Input: part model. Units: mm. Frame: model coordinates. A direction names the side the tool comes from. Coordinates: 2 decimals unless noted, no trailing zeros. Write each loop counter-clockwise with the first axis right and the second up, starting at its lowest first coordinate (ties: lowest second). Pieces come first, ordered by that corner, then holes. Notation, with made-up numbers: (9, 42) - (33, 42) arc R14 cw to (33, 68) - close; hole circle Ø5 at (85, -23). An arc over 180 degrees is marked (long way). Use a Markdown table: item, result. Add a question column.
Q1. Section query A-A (x = 0). Return the cut outline in (y, z) (1 decimal).
Q2. Section query D-D (x = -23). Return the cut outline in (y, z) (3 decimals).
Q3. Section query C-C (y = 50.8). Return the cut outline in (x, z) (1 decimal).
Q4. Set-up query: faces 1 (the face through (13.025, 32.07, 4.696)), 2 (the face through (-45.3, 45.4, 4.7)). Return all of +Z, -Z, +X, -X, +Y, -Y with unobstructed straight access to the full face (end or side cutting, diameter ignored); none if empty.
Q5. Mould query, pull axis X, two halves, no side actions, for faces 3 (the face through (23.315, 55.576, 4.696)), 4 (the face through (-25.72, 25.65, 4.83)), 5 (the face through (-22.812, 55.785, 4.696)). Classes: released by +X, released by -X, zero draft, split by the parting line, or undercut.
Q6. Section query B-B (z = 1.25). Return the cut outline in (x, y) (1 decimal), then the cut area to 3 significant figures.
Q7. Material intervals for probe 1 along Y at (x, z) = (0, 4.5) (1 decimal); probe 2 along X at (y, z) = (-2, 7.25); probe 3 along X at (y, z) = (-3.5, 3.5), sorted ascending. Write a range as from..to.
Q8. Pin query (flat end, axial travel): P1, Ø10, axis at x = 46, y = 6.5, coming from the -Z side; P2, Ø4, axis at x = 17.5, z = 8.5, coming from the +Y side; P3, Ø1.5, axis at x = 10.5, z = 3.5, coming from the +Y side; P4, Ø8.5, axis at x = 0, y = 50.8, coming from the +Z side. Return the tip coordinate at first contact, or that it passes through.
from build123d import *

# Parameters (mm, degrees)
F0_R     = 4.7625
F1_DEPTH = 9.525
F2_R     = 12.7635


with BuildPart() as f1:
    # F0 (on Top) → F1 (new body)
    with BuildSketch(Plane.XY):
        with BuildLine():
            ThreePointArc((-38.331487, -4.728468), (-37.68341, -2.403602), (-37.465, 0))
            ThreePointArc((-37.465, 0), (-48.198471, 13.078772), (-63.119934, 5.103084))
            ThreePointArc((-63.119934, 5.103084), (-55.716337, -12.395638), (-38.331487, -4.728468))
        make_face()
        with Locations((-50.8, 0)):
            Circle(F0_R, mode=Mode.SUBTRACT)
        with BuildLine():
            ThreePointArc((-63.119934, 5.103084), (-48.198471, 13.078772), (-37.465, 0))
            ThreePointArc((-37.465, 0), (-37.68341, -2.403602), (-38.331487, -4.728468))
            Line((-38.331487, -4.728468), (-26.491756, 26.491756))
            ThreePointArc((-26.491756, 26.491756), (-43.329554, 24.833377), (-48.240958, 41.024108))
            Line((-48.240958, 41.024108), (-63.119934, 5.103084))
        make_face()
        with BuildLine():
            ThreePointArc((-41.024108, 48.240958), (-45.350293, 45.350293), (-48.240958, 41.024108))
            ThreePointArc((-48.240958, 41.024108), (-43.329554, 24.833377), (-26.491756, 26.491756))
            ThreePointArc((-26.491756, 26.491756), (-23.601091, 30.817941), (-22.586024, 35.921024))
            ThreePointArc((-22.586024, 35.921024), (-28.512495, 47.008672), (-41.024108, 48.240958))
        make_face()
        with BuildLine():
            ThreePointArc((-22.586024, 35.921024), (-23.601091, 30.817941), (-26.491756, 26.491756))
            Line((-26.491756, 26.491756), (0, 37.465))
            ThreePointArc((0, 37.465), (-13.078772, 48.198471), (-5.103084, 63.119934))
            Line((-5.103084, 63.119934), (-41.024108, 48.240958))
            ThreePointArc((-41.024108, 48.240958), (-28.512495, 47.008672), (-22.586024, 35.921024))
        make_face()
        with BuildLine():
            ThreePointArc((-5.103084, 63.119934), (-13.078772, 48.198471), (0, 37.465))
            ThreePointArc((0, 37.465), (9.429269, 41.370731), (13.335, 50.8))
            ThreePointArc((13.335, 50.8), (11.087647, 58.208529), (5.103084, 63.119934))
            ThreePointArc((5.103084, 63.119934), (0, 64.135), (-5.103084, 63.119934))
        make_face()
        with Locations((0, 50.8)):
            Circle(F0_R, mode=Mode.SUBTRACT)
        with BuildLine():
            ThreePointArc((13.335, 50.8), (9.429269, 41.370731), (0, 37.465))
            Line((0, 37.465), (26.491756, 26.491756))
            ThreePointArc((26.491756, 26.491756), (24.833377, 43.329554), (41.024108, 48.240958))
            Line((41.024108, 48.240958), (5.103084, 63.119934))
            ThreePointArc((5.103084, 63.119934), (11.087647, 58.208529), (13.335, 50.8))
        make_face()
        with BuildLine():
            ThreePointArc((41.024108, 48.240958), (24.833377, 43.329554), (26.491756, 26.491756))
            ThreePointArc((26.491756, 26.491756), (41.024108, 23.601091), (49.256024, 35.921024))
            ThreePointArc((49.256024, 35.921024), (48.999796, 38.522554), (48.240958, 41.024108))
            ThreePointArc((48.240958, 41.024108), (45.350293, 45.350293), (41.024108, 48.240958))
        make_face()
        with BuildLine():
            ThreePointArc((49.256024, 35.921024), (41.024108, 23.601091), (26.491756, 26.491756))
            Line((26.491756, 26.491756), (38.331487, -4.728468))
            ThreePointArc((38.331487, -4.728468), (45.883663, 12.395638), (63.119934, 5.103084))
            Line((63.119934, 5.103084), (48.240958, 41.024108))
            ThreePointArc((48.240958, 41.024108), (48.999796, 38.522554), (49.256024, 35.921024))
        make_face()
        with BuildLine():
            ThreePointArc((63.119934, 5.103084), (45.883663, 12.395638), (38.331487, -4.728468))
            ThreePointArc((38.331487, -4.728468), (53.203602, -13.11659), (64.135, 0))
            ThreePointArc((64.135, 0), (63.878772, 2.601529), (63.119934, 5.103084))
        make_face()
        with Locations((50.8, 0)):
            Circle(F0_R, mode=Mode.SUBTRACT)
    extrude(amount=F1_DEPTH)

    # F2
    f2_edges = [f1.edges().sort_by_distance(p)[0] for p in [
        (-26.491756, 26.491756, 4.7625),
        (0, 37.465, 4.7625),
        (26.491756, 26.491756, 4.7625),
    ]]
    fillet(f2_edges, radius=F2_R)


solid = f1.part
Values follow:
| question | item | result |
|---|---|---|
| 1 | outline | (36.4, 0) - (46, 0) - (46, 9.5) - (36.4, 9.5) - close; (55.6, 0) - (64.1, 0) - (64.1, 9.5) - (55.6, 9.5) - close |
| 2 | outline | (27.802, 0) - (55.707, 0) - (55.707, 9.525) - (27.802, 9.525) - close |
| 3 | outline | (-34.8, 0) - (-4.8, 0) - (-4.8, 9.5) - (-34.8, 9.5) - close; (4.8, 0) - (34.8, 0) - (34.8, 9.5) - (4.8, 9.5) - close |
| 4 | face 1 | +Z, -Z, -Y |
| 4 | face 2 | +Z, -Z, -X, +Y |
| 5 | face 3 | released by +X |
| 5 | face 4 | undercut |
| 5 | face 5 | released by -X |
| 6 | outline | (-63.1, 5.1) arc R13.3 ccw (long way) to (-38.3, -4.7) - (-28.4, 21.3) arc R12.8 cw to (-21.4, 28.6) - (-4.9, 35.4) arc R12.8 cw to (4.9, 35.4) - (21.4, 28.6) arc R12.8 cw to (28.4, 21.3) - (38.3, -4.7) arc R13.3 ccw to (64.1, 0) arc R13.3 ccw to (63.1, 5.1) - (48.2, 41) arc R13.3 ccw to (41, 48.2) - (5.1, 63.1) arc R13.3 ccw to (-5.1, 63.1) - (-41, 48.2) arc R13.3 ccw to (-48.2, 41) - close; hole circle Ø9.5 at (-50.8, 0); hole circle Ø9.5 at (0, 50.8); hole circle Ø9.5 at (50.8, 0) |
| 6 | area | 4,400 mm2 |
| 7 | probe 1 | 36.4..46, 55.6..64.1 |
| 7 | probe 2 | -63.98..-55.12, -46.48..-37.3, 37.3..46.48, 55.12..63.98 |
| 7 | probe 3 | -63.67..-54.03, -47.57..-37.87, 37.87..47.57, 54.03..63.67 |
| 8 | P1 | z = 0 |
| 8 | P2 | y = 58.81 |
| 8 | P3 | y = 61.2 |
| 8 | P4 | through |
